```python
from build123d import *

# Parameters (mm, degrees)
SKETCH1_W                      = 20
SKETCH1_H                      = 60
BASE_FLANGE1_DEPTH             = 2
SKETCH2_R                      = 4
SKETCH2_R_2                    = 1.5
CUT_EXTRUDE1_DEPTH             = 2
EDGE_FLANGE1_STRIP_CUT_DEPTH   = 20
EDGE_FLANGE1_DEPTH             = 20
EDGE_FLANGE2_STRIP_CUT_DEPTH   = 20
EDGE_FLANGE2_DEPTH             = 20
EDGE_FLANGE3_STRIP_CUT_DEPTH   = 20
EDGE_FLANGE3_DEPTH             = 20
EDGE_FLANGE3_START             = 2
EDGE_FLANGE3_FLAT_DEPTH        = 2
EDGE_FLANGE4_STRIP_CUT_DEPTH   = 20
EDGE_FLANGE4_STRIP_CUT_2_DEPTH = 20
EDGE_FLANGE4_DEPTH             = 20
EDGE_FLANGE4_BEND_DEPTH        = 20
SKETCH16_W                     = 5
SKETCH16_H                     = 15
CUT_EXTRUDE2_DEPTH             = 137.190450876
SKETCH23_R                     = 4
SKETCH23_R_2                   = 1.5
CUT_EXTRUDE3_DEPTH             = 10
SKETCH24_R                     = 1.5
CUT_EXTRUDE4_DEPTH             = 10
SKETCH25_R                     = 1.5
CUT_EXTRUDE5_DEPTH             = 10


# Sheet-metal steps are written as plain solids
with BuildPart() as part:
    # Sketch1 → Base-Flange1 (new body)
    with BuildSketch(Plane.XY):
        Rectangle(SKETCH1_W, SKETCH1_H)
    extrude(amount=-BASE_FLANGE1_DEPTH)

    # Sketch2 → Cut-Extrude1 (cut)
    with BuildSketch(Plane.XY):
        with Locations((0, 11)):
            Circle(SKETCH2_R)
        with Locations((0, 18)):
            Circle(SKETCH2_R_2)
        with Locations((7, 11)):
            Circle(SKETCH2_R_2)
        with Locations((0, 4)):
            Circle(SKETCH2_R_2)
        with Locations((-7, 11)):
            Circle(SKETCH2_R_2)
        with Locations(Location((0, -18, 0), (0, 0, 180))):
            Circle(SKETCH2_R_2)
        with Locations(Location((7, -11, 0), (0, 0, 180))):
            Circle(SKETCH2_R_2)
        with Locations(Location((0, -4, 0), (0, 0, 180))):
            Circle(SKETCH2_R_2)
        with Locations(Location((0, -11, 0), (0, 0, 180))):
            Circle(SKETCH2_R)
        with Locations(Location((-7, -11, 0), (0, 0, 180))):
            Circle(SKETCH2_R_2)
    extrude(amount=-CUT_EXTRUDE1_DEPTH, mode=Mode.SUBTRACT)

    # Edge-Flange1 strip (across the edge) → Edge-Flange1 strip cut (cut)
    with BuildSketch(Plane(origin=(-10, 30, -2), x_dir=(0, -0.3420201433256626, -0.9396926207859106), z_dir=(1, 0, 0))):
        Polygon((-5.074988048, 8.095806265), (-1.834962826, -0.80608987), (0.044422416, -0.122049584), (-3.195602806, 8.779846552), align=None)
    extrude(amount=EDGE_FLANGE1_STRIP_CUT_DEPTH, mode=Mode.SUBTRACT)

    # Edge-Flange1 section (across the edge) → Edge-Flange1 (add)
    with BuildSketch(Plane(origin=(-10, 30, -2), x_dir=(0, -0.3420201433256626, -0.9396926207859106), z_dir=(1, 0, 0))):
        with BuildLine():
            Line((-2, 0.129882454), (-2, 33.647346039))
            Line((-2, 33.647346039), (0, 33.647346039))
            Line((0, 33.647346039), (0, 0.129882454))
            ThreePointArc((0, 0.129882454), (0.011190609, 0.001973206), (0.044422416, -0.122049584))
            Line((0.044422416, -0.122049584), (-1.834962826, -0.80608987))
            ThreePointArc((-1.834962826, -0.80608987), (-1.958424897, -0.345323149), (-2, 0.129882454))
        make_face()
    extrude(amount=EDGE_FLANGE1_DEPTH)

    # Edge-Flange2 strip (across the edge) → Edge-Flange2 strip cut (cut)
    with BuildSketch(Plane(origin=(10, -30, -2), x_dir=(0, 0.34202014332566344, -0.9396926207859103), z_dir=(-1, 0, 0))):
        Polygon((-5.074988048, 8.095806265), (-1.834962826, -0.80608987), (0.044422416, -0.122049584), (-3.195602806, 8.779846552), align=None)
    extrude(amount=EDGE_FLANGE2_STRIP_CUT_DEPTH, mode=Mode.SUBTRACT)

    # Edge-Flange2 section (across the edge) → Edge-Flange2 (add)
    with BuildSketch(Plane(origin=(10, -30, -2), x_dir=(0, 0.34202014332566344, -0.9396926207859103), z_dir=(-1, 0, 0))):
        with BuildLine():
            Line((-2, 0.129882454), (-2, 49.647346039))
            Line((-2, 49.647346039), (0, 49.647346039))
            Line((0, 49.647346039), (0, 0.129882454))
            ThreePointArc((0, 0.129882454), (0.011190609, 0.001973206), (0.044422416, -0.122049584))
            Line((0.044422416, -0.122049584), (-1.834962826, -0.80608987))
            ThreePointArc((-1.834962826, -0.80608987), (-1.958424897, -0.345323149), (-2, 0.129882454))
        make_face()
    extrude(amount=EDGE_FLANGE2_DEPTH)

    # Edge-Flange3 strip (across the edge) → Edge-Flange3 strip cut (cut)
    with BuildSketch(Plane(origin=(-10, 61.618162781, -13.508070115), x_dir=(0, -0.6427876096865297, -0.7660444431189862), z_dir=(1, 0, 0))):
        Polygon((-5.074988048, 8.095806265), (-1.834962826, -0.80608987), (0.044422416, -0.122049584), (-3.195602806, 8.779846552), align=None)
    extrude(amount=EDGE_FLANGE3_STRIP_CUT_DEPTH, mode=Mode.SUBTRACT)

    # Edge-Flange3 bend section (across the edge) → Edge-Flange3 (add)
    with BuildSketch(Plane(origin=(-10, 61.618162781, -13.508070115), x_dir=(0, -0.6427876096865297, -0.7660444431189862), z_dir=(1, 0, 0))):
        with BuildLine():
            Line((-2, 0.129882454), (0, 0.129882454))
            ThreePointArc((0, 0.129882454), (0.011190609, 0.001973206), (0.044422416, -0.122049584))
            Line((0.044422416, -0.122049584), (-1.834962826, -0.80608987))
            ThreePointArc((-1.834962826, -0.80608987), (-1.958424897, -0.345323149), (-2, 0.129882454))
        make_face()
    extrude(amount=EDGE_FLANGE3_DEPTH)

    # Edge-Flange3 profile (on flange) → Edge-Flange3 flat (add)
    with BuildSketch(Plane(origin=(0, 61.618162781, -13.508070115), x_dir=(1, 0, 0), z_dir=(0, 0.6427876096865297, 0.7660444431189862)).offset(EDGE_FLANGE3_START)):
        Polygon((10, 0.129882454), (10, 19.823673019), (27.5, 19.823673019), (27.5, 39.823673019), (10, 39.823673019), (10, 59.647346039), (-10, 59.647346039), (-10, 39.823673019), (-27.5, 39.823673019), (-27.5, 19.823673019), (-10, 19.823673019), (-10, 0.129882454), align=None)
    extrude(amount=-EDGE_FLANGE3_FLAT_DEPTH)

    # Edge-Flange4 strip (across the edge) → Edge-Flange4 strip cut (cut)
    with BuildSketch(Plane(origin=(27.5, 92.124866203, -39.106233704), x_dir=(-0.34202014332566305, -0.6040227735550457, -0.7198463103929635), z_dir=(0, -0.7660444431189863, 0.6427876096865295))):
        Polygon((-5.074988048, 8.095806265), (-1.834962826, -0.80608987), (0.044422416, -0.122049584), (-3.195602806, 8.779846552), align=None)
    extrude(amount=EDGE_FLANGE4_STRIP_CUT_DEPTH, mode=Mode.SUBTRACT)

    # Edge-Flange4 strip 2 (across the edge) → Edge-Flange4 strip cut 2 (cut)
    with BuildSketch(Plane(origin=(-27.5, 76.80397734, -26.25048151), x_dir=(0.34202014332566305, -0.6040227735550457, -0.7198463103929635), z_dir=(0, 0.7660444431189863, -0.6427876096865295))):
        Polygon((-5.074988048, 8.095806265), (-1.834962826, -0.80608987), (0.044422416, -0.122049584), (-3.195602806, 8.779846552), align=None)
    extrude(amount=EDGE_FLANGE4_STRIP_CUT_2_DEPTH, mode=Mode.SUBTRACT)

    # Edge-Flange4 section (across the edge) → Edge-Flange4 (add)
    with BuildSketch(Plane(origin=(27.5, 92.124866203, -39.106233704), x_dir=(-0.34202014332566305, -0.6040227735550457, -0.7198463103929635), z_dir=(0, -0.7660444431189863, 0.6427876096865295))):
        with BuildLine():
            Line((-2, 0.129882454), (-2, 19.647346039))
            Line((-2, 19.647346039), (0, 19.647346039))
            Line((0, 19.647346039), (0, 0.129882454))
            ThreePointArc((0, 0.129882454), (0.011190609, 0.001973206), (0.044422416, -0.122049584))
            Line((0.044422416, -0.122049584), (-1.834962826, -0.80608987))
            ThreePointArc((-1.834962826, -0.80608987), (-1.958424897, -0.345323149), (-2, 0.129882454))
        make_face()
    extrude(amount=EDGE_FLANGE4_DEPTH)

    # Edge-Flange4 section 2 (across the edge) → Edge-Flange4 bend (add)
    with BuildSketch(Plane(origin=(-27.5, 76.80397734, -26.25048151), x_dir=(0.34202014332566305, -0.6040227735550457, -0.7198463103929635), z_dir=(0, 0.7660444431189863, -0.6427876096865295))):
        with BuildLine():
            Line((-2, 0.129882454), (-2, 19.647346039))
            Line((-2, 19.647346039), (0, 19.647346039))
            Line((0, 19.647346039), (0, 0.129882454))
            ThreePointArc((0, 0.129882454), (0.011190609, 0.001973206), (0.044422416, -0.122049584))
            Line((0.044422416, -0.122049584), (-1.834962826, -0.80608987))
            ThreePointArc((-1.834962826, -0.80608987), (-1.958424897, -0.345323149), (-2, 0.129882454))
        make_face()
    extrude(amount=EDGE_FLANGE4_BEND_DEPTH)

    # Sketch16 → Cut-Extrude2 (cut, through all)
    with BuildSketch(Plane(origin=(0, -3.55058603, 9.755154944), x_dir=(1, 0, 0), z_dir=(0, -0.3420201433256634, 0.9396926207859103))):
        with Locations((-7.5, -71.022164949)):
            Rectangle(SKETCH16_W, SKETCH16_H)
        with Locations((7.5, -71.022164949)):
            Rectangle(SKETCH16_W, SKETCH16_H)
    extrude(amount=-CUT_EXTRUDE2_DEPTH, mode=Mode.SUBTRACT)

    # Sketch23 → Cut-Extrude3 (cut)
    with BuildSketch(Plane(origin=(0, 20.093289682, 23.946250166), x_dir=(1, 0, 0), z_dir=(0, 0.6427876096865298, 0.7660444431189862))):
        with Locations(Location((0, 96.708744314, 0), (0, 0, 270))):
            Circle(SKETCH23_R)
        with Locations(Location((0, 103.708744314, 0), (0, 0, 270))):
            Circle(SKETCH23_R_2)
        with Locations(Location((7, 96.708744314, 0), (0, 0, 270))):
            Circle(SKETCH23_R_2)
        with Locations(Location((0, 89.708744314, 0), (0, 0, 270))):
            Circle(SKETCH23_R_2)
        with Locations(Location((-7, 96.708744314, 0), (0, 0, 270))):
            Circle(SKETCH23_R_2)
        with Locations(Location((0, 74.708744314, 0), (0, 0, 90))):
            Circle(SKETCH23_R)
        with Locations(Location((7, 74.708744314, 0), (0, 0, 90))):
            Circle(SKETCH23_R_2)
        with Locations(Location((0, 81.708744314, 0), (0, 0, 90))):
            Circle(SKETCH23_R_2)
        with Locations(Location((-7, 74.708744314, 0), (0, 0, 90))):
            Circle(SKETCH23_R_2)
        with Locations(Location((0, 67.708744314, 0), (0, 0, 90))):
            Circle(SKETCH23_R_2)
    extrude(amount=-CUT_EXTRUDE3_DEPTH, mode=Mode.SUBTRACT)

    # Sketch24 → Cut-Extrude4 (cut)
    with BuildSketch(Plane(origin=(-12.620746139, 22.288798586, 26.56275579), x_dir=(-0.9396926207859104, -0.21984631039294733, -0.2620026302293839), z_dir=(0.3420201433256635, -0.6040227735550454, -0.7198463103929638))):
        with Locations(Location((25.690314863, 85.708744314, 0), (0, 0, 90))):
            Circle(SKETCH24_R)
    extrude(amount=-CUT_EXTRUDE4_DEPTH, mode=Mode.SUBTRACT)

    # Sketch25 → Cut-Extrude5 (cut)
    with BuildSketch(Plane(origin=(12.620746139, 22.288798586, 26.56275579), x_dir=(-0.9396926207859105, 0.21984631039294705, 0.26200263022938347), z_dir=(-0.342020143325663, -0.6040227735550456, -0.7198463103929638))):
        with Locations(Location((-25.722785477, 85.708744314, 0), (0, 0, 90))):
            Circle(SKETCH25_R)
    extrude(amount=-CUT_EXTRUDE5_DEPTH, mode=Mode.SUBTRACT)


solid = part.part
```
Source: CAD feature listing. Evaluate the final solid. Frame: model axes, mm. A direction names the side the tool comes from. Coordinates: 2 decimals unless noted, no trailing zeros. Write each loop counter-clockwise with the first axis right and the second up, starting at its lowest first coordinate (ties: lowest second). Pieces come first, ordered by that corner, then holes. Notation, with made-up numbers: (21, 25) - (42, 25) arc R23 cw to (42, 63) - close; hole circle Ø9 at (-1, -34). An arc over 180 degrees is marked (long way). Answer as a JSON object with one key per item and string values.
Q1. Draft query along X for faces 5 (the flat face through (28.987, 76.901, -26.135)), 6 (the flat face through (39.386, 83.159, -34.452)), 7 (the cylindrical face through (0.45, 97.81, -42.55)). Return one class per face: released by +X, released by -X, zero draft, split by the parting line, or undercut.
Ans:
{"face 5": "zero draft", "face 6": "released by +X", "face 7": "undercut"}
Q2. Section query C-C, the plane x = 24.5. Output: boundary loops of the cut face in (y, z), plus the area to 3 significant figures.
Ans:
{"outline": "(76.8, -26.25) - (92.12, -39.11) - (93.41, -37.57) - (78.09, -24.72) - close", "area": "40.0 mm2"}
Q3. First-contact query: pin 1 Ø1.8 at (x, y) = (0, -18) entering from +Z; pin 2 Ø4 at (x, y) = (0, 18) entering from -Z; pin 3 Ø21 at (y, z) = (34.5, -12) entering from -X; pin 4 Ø5.5 at (y, z) = (-71, -16) entering from +X. Flat tips, straight axial feed; report the tip coordinate or a pass-through.
Ans:
{"pin 1": "passes through", "pin 2": "stops at z = -2", "pin 3": "stops at x = -10", "pin 4": "stops at x = 5"}
Q4. Set-up query: faces 1 (the flat face through (-38.958, 81.676, -35.783)), 2 (the flat face through (-0.14, 46.029, -7.834)), 3 (the flat face through (-28.99, 92.22, -38.99)), 4 (the flat face through (-0.383, 86.119, -31.456)). Return all of +Z, -Z, +X, -X, +Y, -Y with unobstructed straight access to the full face (end or side cutting, diameter ignored); none if empty.
Ans:
{"face 1": "-Z, -Y", "face 2": "-Z, +X, -X", "face 3": "-Z, -X, +Y", "face 4": "+Z, +X, -X, +Y"}
Q5. Section query B-B, the plane y = 28. Output: boundary loops of the cut face in (x, z), plus the area to 3 significant figures.
Ans:
{"outline": "(-10, -2) - (10, -2) - (10, 0) - (-10, 0) - close", "area": "40.0 mm2"}
Q6. Section query A-A, the plane z = -4.5. Output: boundary loops of the cut face in (x, y), plus the area to 3 significant figures.
Ans:
{"outline": "(-10, -42.72) - (10, -42.72) - (10, -36.87) - (-10, -36.87) - close; (-10, 36.87) - (10, 36.87) - (10, 42.72) - (-10, 42.72) - close", "area": "234 mm2"}
Q7. Material intervals for line 1 (X direction, y = -11, z = -0.6); line 2 (X direction, y = -18, z = -1.5); line 3 (Z direction, x = -25.5, y = 88), sorted ascending. Write a range as [from, to].
Ans:
{"line 1": "x = [-10, -8.5], [-5.5, -4], [4, 5.5], [8.5, 10]", "line 2": "x = [-10, -1.5], [1.5, 10]", "line 3": "z = [-35.65, -33.03]"}
